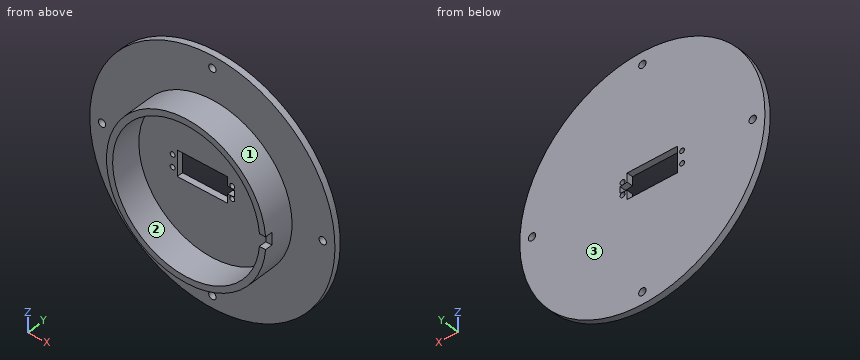
from build123d import *

# Parameters (mm, degrees)
SKETCH_1_R          = 100
EXTRUDE_1_DEPTH     = 5
SKETCH_3_R          = 3
CUT_EXTRUDE_1_DEPTH = 142.509716981
SKETCH_2_R          = 2
SKETCH_2_W          = 41
SKETCH_2_H          = 21
CUT_EXTRUDE_3_DEPTH = 10
SKETCH_4_R          = 65
SKETCH_4_R_2        = 60
EXTRUDE_2_DEPTH     = 25
CUT_EXTRUDE_4_DEPTH = 145.568322948
SKETCH_6_W          = 10
SKETCH_6_H          = 6
CUT_EXTRUDE_5_DEPTH = 165.829829674


with BuildPart() as part:
    # 草图1 → 凸台-拉伸1 (new body)
    with BuildSketch(Plane(origin=(0, 0, 0), x_dir=(1, 0, 0), z_dir=(0, 1, 0))):
        with Locations(Location((0, 0, 0), (0, 0, 270))):
            Circle(SKETCH_1_R)
    extrude(amount=EXTRUDE_1_DEPTH)

    # 草图3 → 切除-拉伸1 (cut, through all)
    with BuildSketch(Plane.XZ):
        with Locations(Location((0, 90, 0), (0, 0, 270))):
            Circle(SKETCH_3_R)
        with Locations(Location((90, 0, 0), (0, 0, 270))):
            Circle(SKETCH_3_R)
        with Locations(Location((0, -90, 0), (0, 0, 270))):
            Circle(SKETCH_3_R)
        with Locations(Location((-90, 0, 0), (0, 0, 270))):
            Circle(SKETCH_3_R)
    extrude(amount=-CUT_EXTRUDE_1_DEPTH, mode=Mode.SUBTRACT)

    # 草图2 → 切除-拉伸3 (cut)
    with BuildSketch(Plane(origin=(0, 0, 0), x_dir=(1, 0, 0), z_dir=(0, 1, 0))):
        with Locations(Location((16.177013134, 5, 0), (0, 0, 270))):
            Circle(SKETCH_2_R)
        with Locations(Location((16.177013134, -5, 0), (0, 0, 90))):
            Circle(SKETCH_2_R)
        with Locations(Location((-32.422986866, -5, 0), (0, 0, 270))):
            Circle(SKETCH_2_R)
        with Locations(Location((-32.422986866, 5, 0), (0, 0, 90))):
            Circle(SKETCH_2_R)
        with Locations((-8.122986866, 0)):
            Rectangle(SKETCH_2_W, SKETCH_2_H)
    extrude(amount=CUT_EXTRUDE_3_DEPTH, mode=Mode.SUBTRACT)

    # 草图4 → 凸台-拉伸2 (add)
    with BuildSketch(Plane.XZ):
        with Locations(Location((0, 0, 0), (0, 0, 270))):
            Circle(SKETCH_4_R)
        with Locations(Location((0, 0, 0), (0, 0, 270))):
            Circle(SKETCH_4_R_2, mode=Mode.SUBTRACT)
    extrude(amount=EXTRUDE_2_DEPTH)

    # 草图5 → 切除-拉伸4 (cut, through all)
    with BuildSketch(Plane(origin=(0, 5, 0), x_dir=(1, 0, 0), z_dir=(0, 1, 0))):
        Polygon((12.377013134, 3.25), (12.377013134, 0), (18.12919557, 0), (18.12919557, 2.6), align=None)
        Polygon((12.377013134, 0), (12.377013134, -3.25), (18.12919557, -2.6), (18.12919557, 0), align=None)
    extrude(amount=-CUT_EXTRUDE_4_DEPTH, mode=Mode.SUBTRACT)

    # 草图6 → 切除-拉伸5 (cut, through all)
    with BuildSketch(Plane(origin=(-28.622986866, 0, 0), x_dir=(0, 0, -1), z_dir=(1, 0, 0))):
        with Locations((0, -22)):
            Rectangle(SKETCH_6_W, SKETCH_6_H)
    extrude(amount=CUT_EXTRUDE_5_DEPTH, mode=Mode.SUBTRACT)


solid = part.part
CAD build for the part. Positions are in the model's coordinates, mm. Face numbers are marked on the shaded views. Coordinates: 2 decimals unless noted, no trailing zeros. Loops run counter-clockwise (first coordinate to the right, second up) from the corner with the lowest first, then second, coordinate; pieces in that order, holes last. Notation, with made-up numbers: (-38, 81.25) - (-23, 81.25) arc R22 ccw to (-23, 90.25) - close; hole circle Ø5 at (61, 58.25). An arc over 180 degrees is marked (long way). Write item = value, one per line. Start each with the question number.
Q1. Drill centre lines: L1, parallel to X at y = 3.75, z = 0; L2, parallel to X at y = 3.7, z = 5; L3, parallel to X at y = -13.25, z = 0. Where is each one in solid material? Low to high.
Q2. Flat gauge pins, fed straight in: pin 1 Ø2 at (x, z) = (1.5, 23) entering from -Y; pin 2 Ø8 at (y, z) = (-11.5, -53.5) entering from -X; pin 3 Ø5 at (y, z) = (-13, -53) entering from +X; pin 4 Ø3.5 at (x, z) = (16.18, 5) entering from -Y. Where does each tip first touch, or does it go through?
Q3. Cut at A-A, the plane z = 0. List the corners of the cut face in (x, y).
Q4. Cut at C-C, the plane x = -90. List the corners of the cut face in (y, z), then the cut area to 3 significant figures.
Q5. Pull direction X, two halves, no side cores. Call the marked faces 1, 2 and 3: pulls with the +X half, pulls with the -X half, needs draft (parallel to the pull), parting line crosses it, or undercut.
Q6. Cut at B-B, the plane x = 0. List the corners of the cut face in (y, z).
Q7. Cut at D-D, the plane y = 2.5. Give the number of separate pieces and of enclosed holes in the cut face, then the cut area to 3 significant figures.
Computed:
q1.L1 = -100 to -93, -87 to -28.62, 18.13 to 87, 93 to 100
q1.L2 = -99.87 to -34.42, -30.42 to -28.62, 12.38 to 14.18, 18.18 to 99.87
q1.L3 = -65 to -60, 60 to 65
q2.pin_1 = 0
q2.pin_2 = -42.13
q2.pin_3 = 40.92
q2.pin_4 = through
q3.outline = (-100, 0) - (-93, 0) - (-93, 5) - (-100, 5) - close; (-87, 0) - (-65, 0) - (-65, -25) - (-60, -25) - (-60, 0) - (-28.62, 0) - (-28.62, 5) - (-87, 5) - close; (18.13, 0) - (60, 0) - (60, -19) - (65, -19) - (65, 0) - (87, 0) - (87, 5) - (18.13, 5) - close; (93, 0) - (100, 0) - (100, 5) - (93, 5) - close
q4.outline = (0, -43.59) - (5, -43.59) - (5, -3) - (0, -3) - close; (0, 3) - (5, 3) - (5, 43.59) - (0, 43.59) - close
q4.area = 406 mm²
q5.face_1 = parting line crosses it
q5.face_2 = undercut
q5.face_3 = needs draft
q6.outline = (-25, -65) - (0, -65) - (0, -87) - (5, -87) - (5, -10.5) - (0, -10.5) - (0, -60) - (-25, -60) - close; (-25, 60) - (0, 60) - (0, 10.5) - (5, 10.5) - (5, 87) - (0, 87) - (0, 65) - (-25, 65) - close; (0, -100) - (5, -100) - (5, -93) - (0, -93) - close; (0, 93) - (5, 93) - (5, 100) - (0, 100) - close
q7.separate_pieces = 1
q7.enclosed_holes = 9
q7.area = 30,400 mm²
